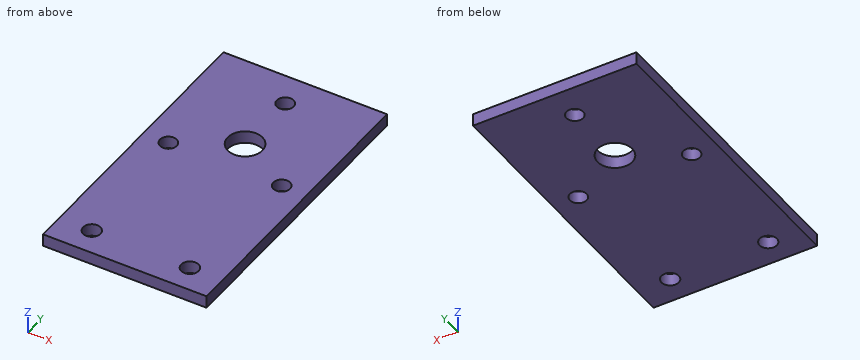
from build123d import *

# Parameters (mm, degrees)
SKETCH1_W                        = 63.5
SKETCH1_H                        = 114.3
BOSS_EXTRUDE1_DEPTH              = 4.826
F_0_257_DIAMETER_HOLE2_D         = 6.7564
F_0_257_DIAMETER_HOLE5_D         = 6.5278
F_17_32_0_53125_DIAMETER_HOLE1_D = 13.49375


with BuildPart() as part:
    # Sketch1 → Boss-Extrude1 (new body)
    with BuildSketch(Plane.XY):
        with Locations((31.75, 57.15)):
            Rectangle(SKETCH1_W, SKETCH1_H)
    extrude(amount=-BOSS_EXTRUDE1_DEPTH)

    # F (0.257) Diameter Hole2 (through all)
    with Locations(Plane.XY):
        with Locations((12.7, 10.16), (50.8, 10.16)):
            Hole(F_0_257_DIAMETER_HOLE2_D / 2)

    # F (0.257) Diameter Hole5 (through all)
    with Locations(Plane.XY):
        with Locations((31.75, 101.6), (9.7536, 63.5), (53.7464, 63.5)):
            Hole(F_0_257_DIAMETER_HOLE5_D / 2)

    # 17/32 (0.53125) Diameter Hole1 (through all)
    with Locations(Plane.XY):
        with Locations((31.75, 76.2)):
            Hole(F_17_32_0_53125_DIAMETER_HOLE1_D / 2)


solid = part.part
Work out the finished part from the listing and answer in its coordinate system (mm). Give positions to 0.01 mm unless a question says otherwise; leave off trailing zeros. Order: outer loops, then holes, each group sorted by start corner. A loop starts at its lowest first (then second) coordinate and runs counter-clockwise, first axis right, second up. Notation, with made-up numbers: M -13.5,-36 L 0.5,-36 A22 cw 0.5,-7 Z; hole C 13,-38.75 d9. An arc over 180 degrees is marked long. Return JSON: item names as keys, results as strings.
Q1. Find section A-A, the plane x = 31.75. Write down the section's boundary in (y, z).
Answer below:
{"outline": "M 0,-4.83 L 69.45,-4.83 L 69.45,0 L 0,0 Z; M 82.95,-4.83 L 98.34,-4.83 L 98.34,0 L 82.95,0 Z; M 104.86,-4.83 L 114.3,-4.83 L 114.3,0 L 104.86,0 Z"}
Q2. Find section C-C, the plane y = 63.5. Write down the section's boundary in (x, z).
Answer below:
{"outline": "M 0,-4.83 L 6.49,-4.83 L 6.49,0 L 0,0 Z; M 13.02,-4.83 L 50.48,-4.83 L 50.48,0 L 13.02,0 Z; M 57.01,-4.83 L 63.5,-4.83 L 63.5,0 L 57.01,0 Z"}
Q3. Find section D-D, the plane z = -2.85. Write down the section's boundary in (x, y), and give its area (3 significant figures).
Answer below:
{"outline": "M 0,0 L 63.5,0 L 63.5,114.3 L 0,114.3 Z; hole C 9.75,63.5 d6.53; hole C 12.7,10.16 d6.76; hole C 31.75,76.2 d13.49; hole C 31.75,101.6 d6.53; hole C 50.8,10.16 d6.76; hole C 53.75,63.5 d6.53", "area": "6,940 mm^2"}
Q4. Find the intervals of material crossed by line 1 along Y through (x, z) = (31.75, -3.2); line 2 along Y through (x, z) = (10, -2.6); line 3 along X through (y, z) = (75, -0.6), in increasing order. Write a range as [from, to].
Answer below:
{"line 1": "y = [0, 69.45], [82.95, 98.34], [104.86, 114.3]", "line 2": "y = [0, 8.13], [12.19, 60.25], [66.75, 114.3]", "line 3": "x = [0, 25.11], [38.39, 63.5]"}
Q5. This flat-tipped pin is pushed along its axis until it touches: pin 1 (17.5 mm diameter, centred on x = 31.75, y = 76.2, fed in from -Z). Where does it stop, or does it pass through?
Answer below:
{"pin 1": "stops at z = -4.83"}
Q6. Find section B-B, the plane y = 76.2. Write down the section's boundary in (x, z), and give its area (3 significant figures).
Answer below:
{"outline": "M 0,-4.83 L 25,-4.83 L 25,0 L 0,0 Z; M 38.5,-4.83 L 63.5,-4.83 L 63.5,0 L 38.5,0 Z", "area": "241 mm^2"}
